from build123d import *

# Parameters (mm, degrees)
CUT_EXTRUDE_1_REACH      = 42.247
CUT_EXTRUDE_1_END_RADIUS = 14.5
SKETCH_2_R               = 3


with BuildPart() as part:
    # Sketch 259 → Повернуть1 (revolve)
    with BuildSketch(Plane.XY, mode=Mode.PRIVATE) as revolve_1_sk:
        with BuildLine():
            Line((0, 6), (22.7, 6))
            Line((22.7, 6), (22.7, 14.5))
            Line((22.7, 14.5), (10.7, 14.5))
            Line((10.7, 14.5), (10.7, 23.5))
            Line((10.7, 23.5), (9, 23.5))
            Line((9, 23.5), (9, 22.49))
            ThreePointArc((9, 22.49), (7.977802666, 20.022197334), (5.51, 19))
            Line((5.51, 19), (5.49, 19))
            ThreePointArc((5.49, 19), (3.022197334, 20.022197334), (2, 22.49))
            Line((2, 22.49), (2, 23.5))
            Line((2, 23.5), (0, 23.5))
            Line((0, 23.5), (0, 6))
        make_face()
    revolve(revolve_1_sk.sketch.rotate(Axis((0, 0, 0), (1, 0, 0)), 90), axis=Axis((0, 0, 0), (1, 0, 0)))

    # Вырез-Вытянуть1: up to this cylinder (the profile starts inside it)
    cut_extrude_1_end = Plane(origin=(16.7, 0, 0), z_dir=(-1, 0, 0)) * Cylinder(CUT_EXTRUDE_1_END_RADIUS, 114.494, mode=Mode.PRIVATE)
    # Эскиз2 → Вырез-Вытянуть1 (cut, up to the surface)
    with BuildSketch(Plane(origin=(0, 0, 0), x_dir=(1, 0, 0), z_dir=(0, 1, 0)), mode=Mode.PRIVATE) as cut_extrude_1_sk1:
        with Locations(Location((16.7, 0, 0), (0, 0, 270))):
            Circle(SKETCH_2_R)
    cut_extrude_1_tool1 = extrude(cut_extrude_1_sk1.sketch, amount=-CUT_EXTRUDE_1_REACH, mode=Mode.PRIVATE) & cut_extrude_1_end
    add(cut_extrude_1_tool1.solids().sort_by_distance((16.7, 0, 0))[0], mode=Mode.SUBTRACT)


solid = part.part
Geometry: final body of the model. Coordinates: model frame, mm. A direction names the side the tool comes from. Give positions to 0.01 mm unless a question says otherwise; leave off trailing zeros. Write each loop counter-clockwise with the first axis right and the second up, starting at its lowest first coordinate (ties: lowest second). Pieces come first, ordered by that corner, then holes. Notation, with made-up numbers: (71.5, -26) -> (130.5, -26) arc R27 cw to (130.5, 4) -> close; hole circle Ø8 at (79, -24). An arc over 180 degrees is marked (long way). Answer in a Markdown table with one row per item.
(1) Section query D-D on x = 14.75. Return loops of the section in (y, z).
Answers below:
| item | result |
|---|---|
| outline | (-14.32, -2.28) arc R14.5 ccw (long way) to (-14.32, 2.28) -> (-5.55, 2.28) arc R6 cw (long way) to (-5.55, -2.28) -> close |
(2) Draft query along X for faces 1 (the flat face through (22.7, -0.2, -6.2)), 2 (the cylindrical face through (9.84, -23.3, -3.06)), 3 (the cylindrical face through (16.8, -9.8, -3)). Return one class per face: +X half, -X half, draft (parallel to the pull), parting line (faces both ways), or undercut.
Answers below:
| item | result |
|---|---|
| face 1 | +X half |
| face 2 | draft |
| face 3 | undercut |
(3) Section query C-C on x = 21. Return loops of the section in (y, z).
Answers below:
| item | result |
|---|---|
| outline | circle Ø29 at (0, 0); hole circle Ø12 at (0, 0) |
(4) Section query B-B on z = 0. State how many separate pieces and enclosed holes the cut face has, then the cut area to 3 significant figures.
Answers below:
| item | result |
|---|---|
| separate pieces | 3 |
| enclosed holes | 0 |
| area | 475 mm^2 |
(5) Set-up query: faces 4 (the flat face through (10.7, -11, -10)), 5 (the flat face through (0, 5, 5)), 6 (the flat face through (9, 0, 23)). Return all of +Z, -Z, +X, -X, +Y, -Y with unobstructed straight access to the full face (end or side cutting, diameter ignored); none if empty.
Answers below:
| item | result |
|---|---|
| face 4 | +X |
| face 5 | +Z, -Z, -X, +Y, -Y |
| face 6 | none |
(6) Ray query, line 1 along Y through (x, z) = (11.25, 0); line 2 along X through (y, z) = (-7.25, 0); line 3 along X through (y, z) = (16, 9.5). Return the intervals inside material, ascending. Write a range as [from, to].
Answers below:
| item | result |
|---|---|
| line 1 | [-14.5, -6], [6, 14.5] |
| line 2 | [0, 13.7], [19.7, 22.7] |
| line 3 | [0, 10.7] |
(7) Pin query (flat end, axial travel): pin 1 (1 mm diameter, centred on x = 9, z = 4.5, fed in from -Y); pin 2 (1 mm diameter, centred on x = 18, z = -12.5, fed in from -Y); pin 3 (3.5 mm diameter, centred on x = 16.7, z = 0, fed in from +Y). Return the tip coordinate at first contact, or that it passes through.
Answers below:
| item | result |
|---|---|
| pin 1 | y = -23.16 |
| pin 2 | y = -8.14 |
| pin 3 | y = 14.5 |
